from build123d import *

# Parameters (mm, degrees)
F1_DEPTH = 35
F2_R     = 2.75
F3_DEPTH = 40


with BuildPart() as f1:
    # F0 (on Right) → F1 (new body)
    with BuildSketch(Plane.YZ):
        with BuildLine():
            Line((40, 0), (0, 0))
            Line((0, 0), (0, -40))
            Line((0, -40), (40, -40))
            Line((40, -40), (40, -39.5))
            ThreePointArc((40, -39.5), (40.146447, -39.146447), (40.5, -39))
            Line((40.5, -39), (109.5, -39))
            ThreePointArc((109.5, -39), (109.853553, -39.146447), (110, -39.5))
            Line((110, -39.5), (110, -40))
            Line((110, -40), (150, -40))
            Line((150, -40), (150, 0))
            Line((150, 0), (110, 0))
            Line((110, 0), (110, -0.5))
            ThreePointArc((110, -0.5), (109.853553, -0.853553), (109.5, -1))
            Line((109.5, -1), (40.5, -1))
            ThreePointArc((40.5, -1), (40.146447, -0.853553), (40, -0.5))
            Line((40, -0.5), (40, 0))
        make_face()
        with BuildLine():
            ThreePointArc((67.5, -16.5), (64.671573, -9.671573), (71.5, -12.5))
            Line((71.5, -12.5), (78.5, -12.5))
            ThreePointArc((78.5, -12.5), (85.328427, -9.671573), (82.5, -16.5))
            Line((82.5, -16.5), (82.5, -23.5))
            ThreePointArc((82.5, -23.5), (85.328427, -30.328427), (78.5, -27.5))
            Line((78.5, -27.5), (71.5, -27.5))
            ThreePointArc((71.5, -27.5), (64.671573, -30.328427), (67.5, -23.5))
            Line((67.5, -23.5), (67.5, -16.5))
        make_face(mode=Mode.SUBTRACT)
    extrude(amount=F1_DEPTH)

    # F2 (on face) → F3 (cut, through all)
    with BuildSketch(Plane.XY):
        with Locations((17.5, 10)):
            Circle(F2_R)
        with Locations((17.5, 30)):
            Circle(F2_R)
        with Locations((25, 20)):
            Circle(F2_R)
        with Locations((10, 20)):
            Circle(F2_R)
        with Locations((17.5, 120)):
            Circle(F2_R)
        with Locations((17.5, 140)):
            Circle(F2_R)
        with Locations((25, 130)):
            Circle(F2_R)
        with Locations((10, 130)):
            Circle(F2_R)
    extrude(amount=-F3_DEPTH, mode=Mode.SUBTRACT)


solid = f1.part
Work out the finished part from the listing and answer in its coordinate system (mm). A direction names the side the tool comes from. Give positions to 0.01 mm unless a question says otherwise; leave off trailing zeros. Loops run counter-clockwise (first coordinate to the right, second up) from the corner with the lowest first, then second, coordinate; pieces in that order, holes last. Notation, with made-up numbers: (72, 62.25) -> (119, 62.25) arc R5 ccw to (119, 67.25) -> close; hole circle Ø2 at (66, 62). An arc over 180 degrees is marked (long way). Use a Markdown table: item, result. Add a question column.
1) The part is cut by section A-A, the plane z = -19. Count the separate pieces of the cut face and the enclosed holes in it, plus the area to 3 significant figures.
2) Consider line 1 along X through (y, z) = (130, -27); line 2 along Y through (x, z) = (8, -14.5); line 3 along Z through (x, y) = (33.5, 82). Determine where each line is inside the solid, lowest interval first.
3) Which of the six approach directions +Z, -Z, +X, -X, +Y, -Y give full straight-line access (tool end or side, diameter ignored) to faces 5 (the flat face through (17, 75, -39)), 6 (the flat face through (17, 75, -1)), 7 (the flat face through (17, 75, -12.5)), 8 (the flat face through (17, 20, 0)), 9 (the cylindrical face through (22.253, 20.121, -19.72))?
4) The part is cut by section C-C, the plane y = 20. Determine the outline of the cut face in (x, z), plus the area to 3 significant figures.
5) For a pull along X with two mould halves and no side action, classify faces 1 (the cylindrical face through (17.255, 64.58, -9.766)), 2 (the cylindrical face through (17.142, 32.727, -19.72)), 3 (the flat face through (35, 74, -11)), 4 (the cylindrical face through (16.904, 117.315, -19.72)) as +X half, -X half, draft (parallel to the pull), parting line (faces both ways), or undercut.
6) Each of these flat-tipped pins is pushed along its axis until it touches: P1, Ø8, axis at x = 20, y = 129, coming from the +Z side; P2, Ø5.5, axis at x = 21.5, y = 74, coming from the -Z side; P3, Ø5.5, axis at x = 13, y = 75.5, coming from the +Z side. Where does it stop, or does it pass through?
Reported:
| question | item | result |
|---|---|---|
| 1 | separate pieces | 2 |
| 1 | enclosed holes | 8 |
| 1 | area | 4,530 mm^2 |
| 2 | line 1 | x = 0 to 7.25, 12.75 to 22.25, 27.75 to 35 |
| 2 | line 2 | y = 0 to 18.11, 21.89 to 64.04, 85.96 to 128.11, 131.89 to 150 |
| 2 | line 3 | z = -39 to -31.47, -8.53 to -1 |
| 3 | face 5 | -Z, +X, -X |
| 3 | face 6 | +Z, +X, -X |
| 3 | face 7 | +X, -X |
| 3 | face 8 | +Z, +X, -X, +Y, -Y |
| 3 | face 9 | +Z, -Z |
| 4 | outline | (0, -40) -> (7.25, -40) -> (7.25, 0) -> (0, 0) -> close; (12.75, -40) -> (22.25, -40) -> (22.25, 0) -> (12.75, 0) -> close; (27.75, -40) -> (35, -40) -> (35, 0) -> (27.75, 0) -> close |
| 4 | area | 960 mm^2 |
| 5 | face 1 | draft |
| 5 | face 2 | undercut |
| 5 | face 3 | +X half |
| 5 | face 4 | undercut |
| 6 | P1 | stops at z = 0 |
| 6 | P2 | stops at z = -39 |
| 6 | P3 | stops at z = -1 |
